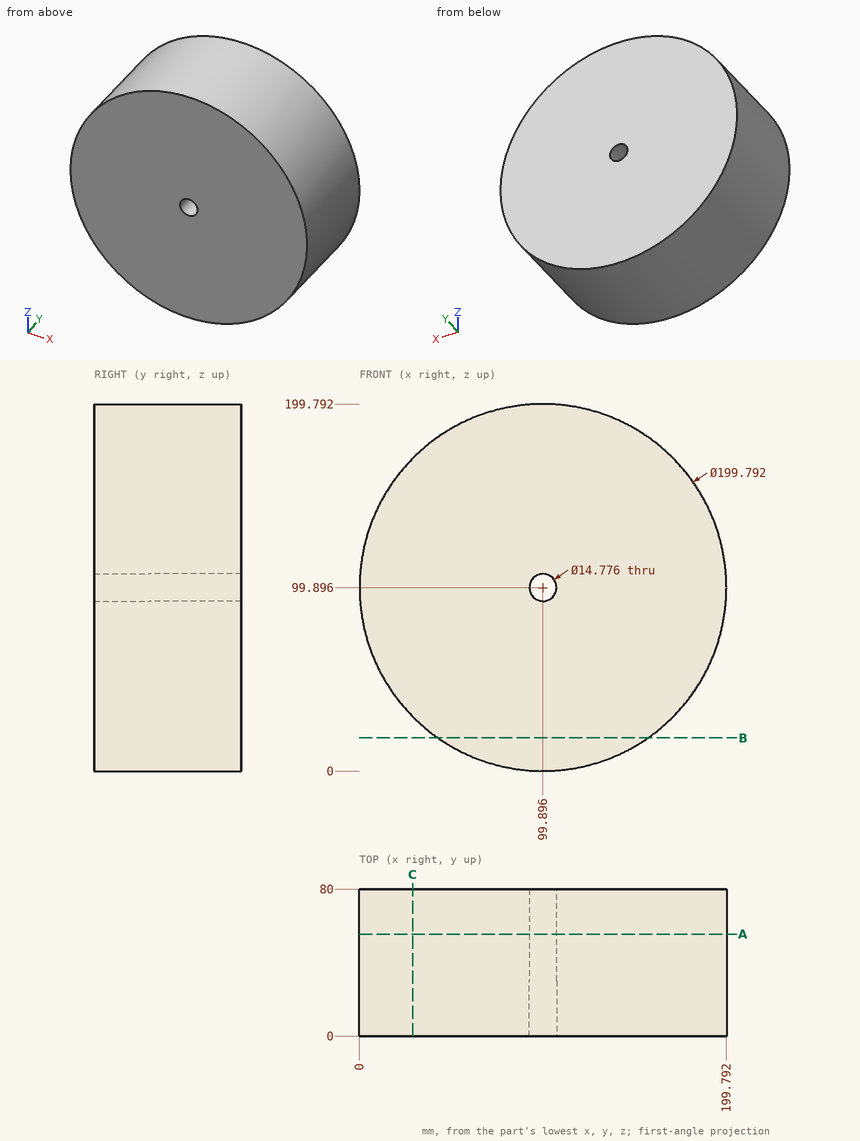
Print and shaded views of the part. All mm, measured from the part's lowest x, y and z. Coordinates: 2 decimals unless noted, no trailing zeros. Write each loop counter-clockwise with the first axis right and the second up, starting at its lowest first coordinate (ties: lowest second). Pieces come first, ordered by that corner, then holes. Notation, with made-up numbers: (-7.75, -33.5) - (23.25, -33.5) arc R24 ccw to (23.25, -19.5) - close; hole circle Ø6 at (-11, 71). An arc over 180 degrees is marked (long way). One line per question, with ' | ' between items. Start each with the question number.
Q1. Pin check, flat tips, straight feed: pin 1 (3 mm diameter, centred on y = 71.5, z = 150.5, fed in from +X); pin 2 (3 mm diameter, centred on x = 128.5, y = 62.5, fed in from +Z) (1 decimal); pin 3 (3 mm diameter, centred on x = 160, y = 53.5, fed in from +Z); pin 4 (1 mm diameter, centred on x = 66, z = 113, fed in from -Y). Stop position of each tip, or through.
Q2. Cut at A-A, the plane y = 55.5. List the corners of the cut face in (x, z) (1 decimal), then the cut area to 3 significant figures.
Q3. Cut at B-B, the plane z = 18. List the corners of the cut face in (x, y).
Q4. Drill centre lines: line 1 (X direction, y = 37.5, z = 100); line 2 (X direction, y = 5, z = 103) (1 decimal); line 3 (Z direction, x = 104.5, y = 56.5) (1 decimal). Where is each one in solid material? Low to high. Write a range as [from, to].
Q5. Cut at C-C, the plane x = 29. List the corners of the cut face in (y, z).
Answer below:
1) pin 1: x = 186.89 | pin 2: z = 196 | pin 3: z = 180.8 | pin 4: y = 0
2) outline: circle Ø199.8 at (99.9, 99.9); hole circle Ø14.8 at (99.9, 99.9) | area: 31,200 mm^2
3) outline: (42.69, 0) - (157.1, 0) - (157.1, 80) - (42.69, 80) - close
4) line 1: [0, 92.51], [107.28, 199.79] | line 2: [0, 93.2], [106.6, 199.7] | line 3: [0.1, 94.1], [105.7, 199.7]
5) outline: (0, 29.52) - (80, 29.52) - (80, 170.27) - (0, 170.27) - close
